Solid Edge part; units mm, degrees
sketch "Sketch1" plane through (0, 0, 0) normal (0, 0, 1) x (1, 0, 0)
  line L0 (-146.05, 139.7) -> (-146.05, -139.7)
  line L1 (-146.05, -139.7) -> (146.05, -139.7)
  line L2 (146.05, -139.7) -> (146.05, 139.7)
  line L3 (146.05, 139.7) -> (-146.05, 139.7)
  dimension "D1" = 146.05
  dimension "D2" = 146.05
extrude "Protrusion1" add sketch "Sketch1" along normal blind 9.525
sketch "Sketch2" plane through (0, 0, 9.525) normal (0, 0, 1) x (1, 0, 0)
  line L0 (-50.8, -139.7) -> (-50.8, 63.5)
  line L1 (-50.8, 63.5) -> (50.8, 63.5)
  line L2 (50.8, 63.5) -> (50.8, -139.7)
  line L3 (50.8, -139.7) -> (-50.8, -139.7)
  dimension "D1" = 50.8
  dimension "D2" = 50.8
extrude "Cutout1" cut sketch "Sketch2" against normal up to next
sketch "Sketch3" plane through (0, 0, 9.525) normal (0, 0, 1) x (1, 0, 0)
  line L0 (146.05, 38.1) -> (146.05, -38.1)
  line L1 (146.05, -38.1) -> (127, -38.1)
  line L2 (127, -38.1) -> (127, 38.1)
  line L3 (127, 38.1) -> (146.05, 38.1)
  line L4 (-146.05, 38.1) -> (-146.05, -38.1)
  line L5 (-146.05, -38.1) -> (-127, -38.1)
  line L6 (-127, -38.1) -> (-127, 38.1)
  line L7 (-127, 38.1) -> (-146.05, 38.1)
  dimension "D1" = 127
  dimension "D2" = 127
  dimension "D3" = 127
extrude "Cutout2" cut sketch "Sketch3" against normal up to next
sketch "Sketch4" plane through (0, 0, 9.525) normal (0, 0, 1) x (1, 0, 0)
  line L0 (136.525, 101.6) -> (-136.525, 101.6)
  line L1 (-136.525, 139.7) -> (-136.525, 101.6)
  line L2 (136.525, 139.7) -> (-136.525, 139.7)
  line L3 (136.525, 139.7) -> (136.525, 101.6)
  line L4 (79.375, -139.7) -> (79.375, 63.5)
  line L5 (146.05, 63.5) -> (79.375, 63.5)
  line L6 (146.05, 63.5) -> (146.05, 38.1)
  line L7 (146.05, 38.1) -> (127, 38.1)
  line L8 (127, -38.1) -> (127, 38.1)
  line L9 (146.05, -38.1) -> (127, -38.1)
  line L10 (146.05, -38.1) -> (146.05, -139.7)
  line L11 (146.05, -139.7) -> (79.375, -139.7)
  line L12 (-69.85, 63.5) -> (-69.85, -139.7)
  line L13 (-69.85, -139.7) -> (69.85, -139.7)
  line L14 (69.85, -139.7) -> (69.85, 63.5)
  line L15 (69.85, 63.5) -> (-69.85, 63.5)
  line L16 (-79.375, -139.7) -> (-79.375, 63.5)
  line L17 (-146.05, 63.5) -> (-79.375, 63.5)
  line L18 (-146.05, 63.5) -> (-146.05, 38.1)
  line L19 (-146.05, 38.1) -> (-127, 38.1)
  line L20 (-127, -38.1) -> (-127, 38.1)
  line L21 (-146.05, -38.1) -> (-127, -38.1)
  line L22 (-146.05, -38.1) -> (-146.05, -139.7)
  line L23 (-146.05, -139.7) -> (-79.375, -139.7)
  dimension "D1" = 69.85
extrude "Cutout3" cut sketch "Sketch4" against normal through all
hole "Hole_1" at (-74.6125, -76.2, 9.525) direction (0, 0, -1) diameter 4.826 end up to next countersink diameter 9.525 countersink angle 82
hole "Hole1" at (74.6125, -76.2, 9.525) direction (0, 0, -1) diameter 4.826 end up to next countersink diameter 9.525 countersink angle 82
hole "Hole2" at (74.6125, 12.7, 9.525) direction (0, 0, -1) diameter 4.826 end up to next countersink diameter 9.525 countersink angle 82
hole "Hole3" at (-74.6125, 12.7, 9.525) direction (0, 0, -1) diameter 4.826 end up to next countersink diameter 9.525 countersink angle 82
sketch "Sketch5" plane through (0, 0, 9.525) normal (0, 0, 1) x (1, 0, 0)
  line L0 (120.65, 25.4) -> (120.65, -25.4)
  line L1 (120.65, -25.4) -> (79.375, -25.4)
  line L2 (79.375, -25.4) -> (79.375, 25.4)
  line L3 (79.375, 25.4) -> (120.65, 25.4)
  line L4 (-120.65, 25.4) -> (-120.65, -25.4)
  line L5 (-120.65, -25.4) -> (-79.375, -25.4)
  line L6 (-79.375, -25.4) -> (-79.375, 25.4)
  line L7 (-79.375, 25.4) -> (-120.65, 25.4)
  dimension "D1" = 120.65
  dimension "D2" = 120.65
extrude "ExtrudedProtrusion_2" add sketch "Sketch5" against normal blind 9.525
hole "Hole4" at (141.2875, 127, 9.525) direction (0, 0, -1) diameter 4.826 end up to next countersink diameter 9.525 countersink angle 82
hole "Hole5" at (-141.2875, 127, 9.525) direction (0, 0, -1) diameter 4.826 end up to next countersink diameter 9.525 countersink angle 82
fillet "Round_1" radius 19.05 10 edges at (-79.375, 63.5, 4.7625) (-79.375, 25.4, 4.7625) (-79.375, -25.4, 4.7625) (-136.525, 101.6, 4.7625) (136.525, 101.6, 4.7625) (-69.85, 63.5, 4.7625) (69.85, 63.5, 4.7625) (79.375, 63.5, 4.7625) (79.375, 25.4, 4.7625) (79.375, -25.4, 4.7625)
sketch "Sketch6" plane through (0, 44.45, 9.525) normal (0, 0, 1) x (1, 0, 0)
  line L0 (-79.375, -184.15) -> (79.375, -184.15)
  line L1 (79.375, -184.15) -> (79.375, -152.4)
  line L2 (79.375, -152.4) -> (-79.375, -152.4)
  line L3 (-79.375, -152.4) -> (-79.375, -184.15)
  dimension "D1" = 79.375
extrude "ExtrudedCutout_6" cut sketch "Sketch6" against normal blind 63.5
sketch "Sketch7" plane through (0, 6.35, 9.525) normal (0, 0, 1) x (1, 0, 0)
  line L0 (-120.65, 57.15) -> (-120.65, 19.05)
  line L1 (-120.65, 19.05) -> (-75.6751, 19.05)
  line L2 (-75.6751, 19.05) -> (-75.6751, 57.15)
  line L3 (-75.6751, 57.15) -> (-120.65, 57.15)
  line L4 (120.65, 57.15) -> (120.65, 19.05)
  line L5 (120.65, 19.05) -> (75.6751, 19.05)
  line L6 (75.6751, 19.05) -> (75.6751, 57.15)
  line L7 (75.6751, 57.15) -> (120.65, 57.15)
extrude "ExtrudedProtrusion_4" add sketch "Sketch7" against normal blind 9.525
hole "Hole6" at (-74.6125, -88.4555, 9.525) direction (0, 0, -1) diameter 1.6942 end through all
hole "Hole7" at (74.6125, -103.1875, 9.525) direction (0, 0, -1) diameter 1.6942 end through all
hole "Hole8" at (74.6125, -88.4555, 9.525) direction (0, 0, -1) diameter 1.6942 end through all
hole "Hole9" at (-74.6125, -103.1875, 9.525) direction (0, 0, -1) diameter 1.6942 end through all
hole "Hole10" at (-141.2875, 119.634, 9.525) direction (0, 0, -1) diameter 1.6942 end through all
hole "Hole11" at (-141.2875, 134.366, 9.525) direction (0, 0, -1) diameter 1.6942 end through all
hole "Hole12" at (141.2875, 119.634, 9.525) direction (0, 0, -1) diameter 1.6942 end through all
hole "Hole13" at (141.2875, 134.366, 9.525) direction (0, 0, -1) diameter 1.6942 end through all
hole "Hole14" at (-120.65, 17.4625, 4.7625) direction (1, 0, 0) diameter 3.9675 depth 19.05
hole "Hole15" at (-120.65, -17.4625, 4.7625) direction (1, 0, 0) diameter 3.9675 depth 19.05
hole "Hole16" at (120.65, 17.4625, 4.7625) direction (-1, 0, 0) diameter 3.9675 depth 19.05
hole "Hole17" at (120.65, -17.4625, 4.7625) direction (-1, 0, 0) diameter 3.9675 depth 19.05
properties part number "CHAS-01" material "Polyethylene, low density"
Geometry check sheet. Reference: the model listing, model coordinates, mm. A direction names the side the tool comes from. Give positions to 0.01 mm unless a question says otherwise; leave off trailing zeros. Order: outer loops, then holes, each group sorted by start corner. A loop starts at its lowest first (then second) coordinate and runs counter-clockwise, first axis right, second up.
1) Material ranges on probe 1 along X at (y, z) = (-77, 1.75) (3 decimals); probe 2 along X at (y, z) = (-69.5, 1.25) (3 decimals); probe 3 along Y at (x, z) = (102, 6), recorded low to high.
Results are:
probe 1: x = -79.375 to -76.889, -72.336 to -69.85, 69.85 to 72.336, 76.889 to 79.375
probe 2: x = -79.375 to -69.85, 69.85 to 79.375
probe 3: y = -25.4 to -19.01, -15.91 to 15.91, 19.01 to 101.6
2) Cross-section at B-B (x = -57.5). Record the boundary of the cut face in (y, z) (1 decimal).
Results are:
outline: (62.3, 0) - (101.6, 0) - (101.6, 9.5) - (62.3, 9.5) - close
3) Tool access check on faces 1 (the flat face through (69.85, -33, 5)), 2 (the flat face through (120.65, 20, 5)), 3 (the cylindrical face through (-130.797, 107.032, 4.696)). Record the directions out of +Z, -Z, +X, -X, +Y, -Y that give a thin tool (end or side, any length) a straight path to the whole face; none if there is none.
Results are:
face 1: +Z, -Z, -Y
face 2: +Z, -Z, +X, -Y
face 3: +Z, -Z, +Y
4) Cross-section at A-A (y = 35). Record the boundary of the cut face in (x, z) (3 decimals).
Results are:
outline: (-120.65, 0) - (-69.85, 0) - (-69.85, 9.525) - (-120.65, 9.525) - close; (69.85, 0) - (120.65, 0) - (120.65, 9.525) - (69.85, 9.525) - close
5) Gauge pin test, flat ends, axial feed: pin 1 (6.5 mm diameter, centred on x = 74.61, y = 12.7, fed in from +Z); pin 2 (5 mm diameter, centred on y = 17.46, z = 4.76, fed in from -X); pin 3 (2 mm diameter, centred on y = 18, z = 4, fed in from +X). Record the tip position at first contact, or that the pin passes through.
Results are:
pin 1: stops at z = 7.79
pin 2: stops at x = -120.65
pin 3: stops at x = 101.6
6) Draft check along X on faces 4 (the flat face through (1, 63.5, 5)), 5 (the flat face through (75, -92, 9.525)), 6 (the flat face through (-146.05, 102, 5)). Enter one of: released by +X, released by -X, zero draft, split by the parting line, or undercut.
Results are:
face 4: undercut
face 5: zero draft
face 6: released by -X
